Part model, mm, in its own coordinate system. Face numbers are marked on the shaded views. A direction names the side the tool comes from. Round coordinates to 2 decimals unless told otherwise and drop trailing zeros. Write each loop counter-clockwise with the first axis right and the second up, starting at its lowest first coordinate (ties: lowest second). Pieces come first, ordered by that corner, then holes.
1) Saw through at C-C on z = 276.5. Write the cut outline in (x, y).
2) Drill centre lines: L1, parallel to Z at x = 403, y = -124.5; L2, parallel to X at y = -106, z = 246; L3, parallel to Y at x = 145.5, z = 419. Where is each one in solid material? Low to high.
3) Saw through at B-B on x = 259. Write the cut outline in (y, z).
4) Pull direction X, two halves, no side cores. Call the marked faces 3, 4 and 5: +X half, -X half, draft (parallel to the pull), parting line (faces both ways), or undercut.
5) Saw through at A-A on y = -201. Write the cut outline in (x, z).
6) Flat gauge pins, fed straight in: pin 1 (4 mm diameter, centred on x = 604.5, z = 124.5, fed in from -Y); pin 2 (1 mm diameter, centred on x = 609.5, z = 110, fed in from +Y). Where does each tip first touch, or does it go through?
7) Which spindle directions (+Z, -Z, +X, -X, +Y, -Y) get a long thin tool onto all of the face, cutting with end or side? Do the marked faces 1 and 2. Say none if no direction does.
```python
from build123d import *

# Parameters (mm, degrees)
F0_W     = 736.6
F0_H     = 457.2
F2_DEPTH = 219.202
F3_T     = -2.54
F1_W     = 736.6
F1_H     = 457.2
F4_DEPTH = 16.002


with BuildPart() as f2:
    # F0 (on Front) → F2 (new body)
    with BuildSketch(Plane.XZ):
        with Locations((368.3, 228.6)):
            Rectangle(F0_W, F0_H)
    extrude(amount=F2_DEPTH)

    # F3
    f3_openings = [f2.faces().sort_by_distance(p)[0] for p in [
        (368.3, -219.202, 228.6),
    ]]
    offset(amount=F3_T, openings=f3_openings)

    # F1 (on Front) → F4 (join)
    with BuildSketch(Plane.XZ):
        with Locations((368.3, 228.6)):
            Rectangle(F1_W, F1_H)
    extrude(amount=F4_DEPTH)


solid = f2.part
```
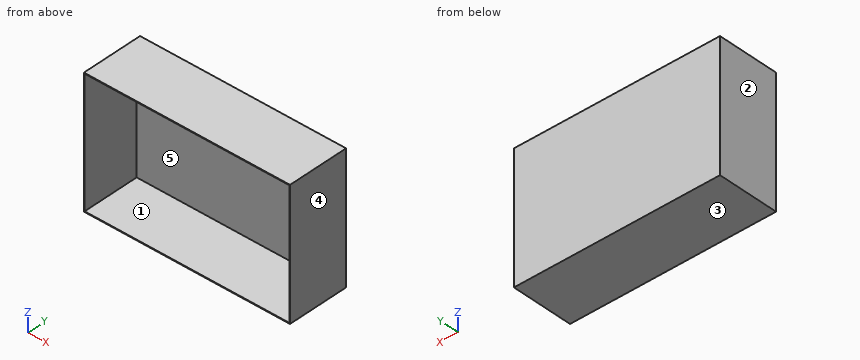
Completed:
1. outline: (0, -219.2) - (2.54, -219.2) - (2.54, -16) - (734.06, -16) - (734.06, -219.2) - (736.6, -219.2) - (736.6, 0) - (0, 0) - close
2. L1: z = 0 to 2.54, 454.66 to 457.2
2. L2: x = 0 to 2.54, 734.06 to 736.6
2. L3: y = -16 to 0
3. outline: (-219.2, 0) - (0, 0) - (0, 457.2) - (-219.2, 457.2) - (-219.2, 454.66) - (-16, 454.66) - (-16, 2.54) - (-219.2, 2.54) - close
4. face 3: draft
4. face 4: +X half
4. face 5: undercut
5. outline: (0, 0) - (736.6, 0) - (736.6, 457.2) - (0, 457.2) - close; hole (2.54, 2.54) - (734.06, 2.54) - (734.06, 454.66) - (2.54, 454.66) - close
6. pin 1: stops at y = -16
6. pin 2: stops at y = 0
7. face 1: -Y
7. face 2: +Z, -Z, -X, +Y, -Y
